```python
from build123d import *

# Parameters (mm, degrees)
SKETCH1_R           = 0.9
BOSS_EXTRUDE1_DEPTH = 7
SKETCH2_R           = 2.5
BOSS_EXTRUDE2_DEPTH = 1
DOME1_FACE_RADIUS   = 2.5
DOME1_HEIGHT        = 0.5
SKETCH3_W           = 1.125
SKETCH3_H           = 0.75
SKETCH3_W_2         = 0.75
SKETCH3_H_2         = 1.125
CUT_EXTRUDE1_DEPTH  = 0.75


with BuildPart() as part:
    # Sketch1 → Boss-Extrude1 (new body)
    with BuildSketch(Plane(origin=(0, 0, 0), x_dir=(1, 0, 0), z_dir=(0, 1, 0))):
        Circle(SKETCH1_R)
    extrude(amount=BOSS_EXTRUDE1_DEPTH)

    # Sketch2 → Boss-Extrude2 (add)
    with BuildSketch(Plane(origin=(0, 7, 0), x_dir=(1, 0, 0), z_dir=(0, 1, 0))):
        Circle(SKETCH2_R)
    extrude(amount=BOSS_EXTRUDE2_DEPTH)

    # Dome1: a dome of height H over a round flat face of radius A is a cap of a sphere of radius (A * A + H * H) / (2 * H)
    dome1_r = (DOME1_FACE_RADIUS * DOME1_FACE_RADIUS + DOME1_HEIGHT * DOME1_HEIGHT) / (2 * DOME1_HEIGHT)
    dome1_base = Plane((0, 8, 0), z_dir=(0, 1, 0))
    with Locations(dome1_base.offset(DOME1_HEIGHT - dome1_r)):
        dome1_ball = Sphere(dome1_r, mode=Mode.PRIVATE)
    add(split(dome1_ball, bisect_by=dome1_base, keep=Keep.TOP, mode=Mode.PRIVATE))

    # Sketch3 → Cut-Extrude1 (cut)
    with BuildSketch(Plane(origin=(0, 8.5, 0), x_dir=(1, 0, 0), z_dir=(0, 1, 0))):
        with Locations((-0.9375, 0)):
            Rectangle(SKETCH3_W, SKETCH3_H)
        Rectangle(SKETCH3_W_2, SKETCH3_H)
        with Locations((0, 0.9375)):
            Rectangle(SKETCH3_W_2, SKETCH3_H_2)
        with Locations((0.9375, 0)):
            Rectangle(SKETCH3_W, SKETCH3_H)
        with Locations((0, -0.9375)):
            Rectangle(SKETCH3_W_2, SKETCH3_H_2)
    extrude(amount=-CUT_EXTRUDE1_DEPTH, mode=Mode.SUBTRACT)


solid = part.part
```
Verification items for the finished model (mm, model axes). Give positions to 0.01 mm unless a question says otherwise; leave off trailing zeros. Order: outer loops, then holes, each group sorted by start corner. A loop starts at its lowest first (then second) coordinate and runs counter-clockwise, first axis right, second up. Notation, with made-up numbers: M -15,80 L 36,80 A13 cw 36,92 Z; hole C 57,0 d2. An arc over 180 degrees is marked long. Answer in a Markdown table with one row per item. Add a question column.
Item 1: Section check B-B, the plane x = 0. Enter the section's corners in (y, z), and give its area (3 significant figures).
Item 2: Section check D-D, the plane z = -1. Enter the section's corners in (x, y) (3 decimals).
Item 3: Mould release check, pull along X, two halves, no side actions. Record for faces 1 (the flat face through (0, 7, 1.1)), 2 (the cylindrical face through (0.86, 3.45, -0.27)), 3 (the flat face through (0, 7.75, 0)): released by +X, released by -X, zero draft, split by the parting line, or undercut.
Item 4: Gauge pin test, flat ends, axial feed: pin 1 (0.8 mm diameter, centred on y = 8, z = -1, fed in from +X); pin 2 (1.5 mm diameter, centred on x = 0.5, z = 0.5, fed in from +Y); pin 3 (0.6 mm diameter, centred on x = -1, y = 8, fed in from +Z); pin 4 (2 mm diameter, centred on x = 2, z = 0.5, fed in from -Y). Record the tip position at first contact, or that the pin passes through.
Item 5: Scan lines: probe 1 along Y at (x, z) = (-0.1, 1.45); probe 2 along Z at (x, y) = (0.55, 1); probe 3 along X at (y, z) = (4, -0.6). Record each from-to range of solid material in increasing order. Write a range as from..to.
Item 6: Section check A-A, the plane z = 0. Enter the section's corners in (x, y), and give its area (3 significant figures).
Item 7: Section check C-C, the plane y = 7.5. Enter the section's corners in (x, z).
Filled sheet:
| question | item | result |
|---|---|---|
| 1 | outline | M 0,-0.9 L 7,-0.9 L 7,-2.5 L 8,-2.5 A6.5 ccw 8.32,-1.5 L 7.75,-1.5 L 7.75,1.5 L 8.32,1.5 A6.5 ccw 8,2.5 L 7,2.5 L 7,0.9 L 0,0.9 Z |
| 1 | area | 17.2 mm^2 |
| 2 | outline | M -2.291,7 L 2.291,7 L 2.291,8 A6.423 ccw 0.375,8.412 L 0.375,7.75 L -0.375,7.75 L -0.375,8.412 A6.423 ccw -2.291,8 Z |
| 3 | face 1 | zero draft |
| 3 | face 2 | split by the parting line |
| 3 | face 3 | undercut |
| 4 | pin 1 | stops at x = 2.43 |
| 4 | pin 2 | stops at y = 8.48 |
| 4 | pin 3 | stops at z = 2.4 |
| 4 | pin 4 | stops at y = 7 |
| 5 | probe 1 | y = 7..7.75 |
| 5 | probe 2 | z = -0.71..0.71 |
| 5 | probe 3 | x = -0.67..0.67 |
| 6 | outline | M -2.5,7 L -0.9,7 L -0.9,0 L 0.9,0 L 0.9,7 L 2.5,7 L 2.5,8 A6.5 ccw 1.5,8.32 L 1.5,7.75 L -1.5,7.75 L -1.5,8.32 A6.5 ccw -2.5,8 Z |
| 6 | area | 17.2 mm^2 |
| 7 | outline | C 0,0 d5 |
